Autodesk Inventor part; units mm, degrees
ref_plane "Work Plane2" through (0, 0, 20.5) normal (0, 0, 1) x (1, 0, 0)
ref_plane "YZ Plane" through (0, 0, 0) normal (1, 0, 0) x (0, 1, 0)
ref_plane "XZ Plane" through (0, 0, 0) normal (0, 1, 0) x (-1, 0, 0)
sketch "Sketch1" plane through (0, 0, 0) normal (0, 0, 1) x (1, 0, 0)
  circle A0 centre (0, 0) radius 20
  circle A1 centre (0, 15.55) radius 1.6
  line L0 (-20, 0) -> (20, 0) construction
  line L1 (20, 0) -> (20, -42)
  line L2 (20, -42) -> (-20, -42)
  line L3 (-20, -42) -> (-20, 0)
  circle A2 centre (-13.4667, 7.775) radius 1.6
  circle A3 centre (-13.4667, -7.775) radius 1.6
  circle A4 centre (0, -15.55) radius 1.6
  circle A5 centre (13.4667, -7.775) radius 1.6
  circle A6 centre (13.4667, 7.775) radius 1.6
  line L4 (0, -7) -> (0, 7) construction
  line L5 (-6.5, -7) -> (-6.5, 7)
  line L6 (6.5, 7) -> (6.5, -7)
  arc A7 (-6.5, -7) -> (6.5, -7) centre (0, -7) ccw
  arc A8 (6.5, 7) -> (-6.5, 7) centre (0, 7) ccw
  dimension "d0" = 40
  dimension "d1" = 15.55
  dimension "d3" = 42
  dimension "d6" = 360
  dimension "d8" = 6.5
  dimension "d9" = 14
extrude "Extrusion1" add sketch "Sketch1" along normal blind 7 contours A0 | L1 L2 L3 A0 | A1 | A2 | A3 | A4 | A5 | A6
sketch "Sketch2" plane through (0, 0, 0) normal (0, 0, -1) x (-1, 0, 0)
  line L0 (20, 0) -> (20, -42)
  arc A0 (20, 0) -> (-20, 0) centre (0, 0) ccw
  line L1 (-20, -42) -> (-20, 0)
  line L2 (20, -42) -> (-20, -42)
  line L3 (-6.5, 7) -> (-6.5, -7)
  arc A1 (6.5, 7) -> (-6.5, 7) centre (0, 7) ccw
  line L4 (6.5, -7) -> (6.5, 7)
  arc A2 (-6.5, -7) -> (6.5, -7) centre (0, -7) ccw
  circle A3 centre (0, 0) radius 15.5 construction
  circle A4 centre (-7.75, 13.4234) radius 1.6
  line L5 (0, 0) -> (-7.75, 13.4234) construction
  line L6 (0, 0) -> (0, 15.5) construction
  circle A5 centre (-15.5, 0) radius 1.6
  circle A6 centre (-7.75, -13.4234) radius 1.6
  circle A7 centre (7.75, -13.4234) radius 1.6
  circle A8 centre (15.5, 0) radius 1.6
  circle A9 centre (7.75, 13.4234) radius 1.6
  dimension "d12" = 31
  dimension "d13" = 3.2
  dimension "d14" = 30
  dimension "d17" = 360
extrude "Extrusion2" cut sketch "Sketch2" against normal through all contours A4 | A5 | A6 | A7 | A8 | A9
sketch "Sketch3" plane through (-20, -42, 0) normal (0, -1, 0) x (1, 0, 0)
  line L0 (0, 0) -> (40, 0)
  line L1 (40, 0) -> (40, 7)
  line L2 (0, 7) -> (40, 7)
  line L3 (0, 0) -> (0, 7)
  line L4 (40, 0) -> (40, 7)
  line L5 (40, 7) -> (0, 7)
  line L6 (0, 7) -> (0, 40)
  line L7 (0, 40) -> (40, 40)
  line L8 (40, 40) -> (40, 7)
  point P0 (20, 0)
  dimension "d21" = 40
extrude "Extrusion3" add sketch "Sketch3" against normal blind 8 contours L6 L7 L8 L2
fillet "Fillet1" radius 2 1 edges at (0, -42, 0)
sketch "Sketch4" plane through (-20, -42, 2) normal (0, -1, 0) x (1, 0, 0)
  line L0 (40, 38) -> (0, 38)
  line L1 (0, 0) -> (0, 38)
  line L2 (40, 0) -> (0, 0)
  line L3 (40, 0) -> (40, 38)
  line L4 (5, 4) -> (-5, 4)
  line L5 (-5, 4) -> (-5, 11)
  line L6 (-5, 11) -> (5, 11)
  line L7 (5, 11) -> (5, 4)
  line L8 (5, 4) -> (-5, 11) construction
  line L9 (-5, 4) -> (5, 11) construction
  circle A0 centre (-5, 7.5) radius 3.5
  circle A1 centre (-5, 7.5) radius 1.75
  point P0 (20, -2)
  point P1 (0, 7.5)
  point P2 (0, 4)
  point P3 (0, 11)
  point P4 (-5, 11)
  dimension "d26" = 7
  dimension "d27" = 5
  dimension "d28" = 4
  dimension "d29" = 3.5
extrude "Extrusion4" add sketch "Sketch4" against normal blind 4 contours L1 L4 A0 L6 | A0 L5 A1 | L5 A1 A0
ref_plane "Work Plane1" through (0, 0, 22.5) normal (0, 0, 1) x (1, 0, 0)
ref_plane "Work Plane2" through (0, 0, 20.5) normal (0, 0, 1) x (1, 0, 0)
mirror "Mirror2" about plane through (0, 0, 0) normal (1, 0, 0) of "Extrusion4"
mirror "Mirror3" about plane through (0, 0, 20.5) normal (0, 0, 1) of "Extrusion4", "Mirror2"
fillet "Fillet4" radius 2 8 edges at (20, -40, 6) (20, -40, 28) (-20, -40, 6) (-20, -40, 13) (-20, -40, 28) (-20, -40, 35) (20, -40, 35) (20, -40, 13)
properties part number "08_Ga_dong_co_02" material "Polyethylene, High Density"
Geometry check sheet. Reference: the model listing, model coordinates, mm. A direction names the side the tool comes from. Coordinates: 2 decimals unless noted, no trailing zeros. Loops run counter-clockwise (first coordinate to the right, second up) from the corner with the lowest first, then second, coordinate; pieces in that order, holes last.
Item 1: Access from +Z, -Z, +X, -X, +Y, -Y to the whole of each face (thin tool, end or side, straight path). Record for faces 4 (the face through (-5, -13, 7)), 5 (the face through (24, -40, 6)), 6 (the face through (0.1, -13.5, 3.5)), 7 (the face through (-20, -27.3, 6.6)).
Item 2: Sectioned sample at A-A, the plane z = 31.5. Record the boundary of the cut face in (x, y), then the cut area to 3 significant figures.
Item 3: Sectioned sample at C-C, the plane x = -7.75. Record the boundary of the cut face in (y, z), then the cut area to 3 significant figures.
Item 4: Release check for a two-part mould opening along Z. For faces 1 (the face through (23, -38, 10)), 2 (the face through (26.75, -40.03, 9.42)), 3 (the face through (-23, -40, 6)) record: released by +Z, released by -Z, zero draft, split by the parting line, or undercut.
Item 5: Sectioned sample at D-D, the plane y = -32.5. Record the boundary of the cut face in (x, z), then the cut area to 3 significant figures.
Item 6: Thickness scan on line 1 (X direction, y = -39.4, z = 9.5); line 2 (Z direction, x = 25, y = -39); line 3 (Y direction, x = 7.75, z = 2.5). Record the ranges inside material, lowest first.
Item 7: Go/stop test with flat-tipped pins: pin 1 Ø1 at (x, z) = (-4, 10) entering from +Y; pin 2 Ø8 at (y, z) = (-35, 23.5) entering from +X; pin 3 Ø4 at (x, z) = (-23.5, 11.5) entering from +Y. Record where each tip stops, or that it passes through.
Item 8: Sectioned sample at B-B, the plane x = 0. Record the boundary of the cut face in (y, z).
Check result:
1. face 4: +Z, +X, -X, +Y
1. face 5: -Z, +X, +Y, -Y
1. face 6: +Z, -Z
1. face 7: -X, +Y
2. outline: (-28.5, -42) - (-26.75, -42) - (-26.75, -38) - (-28.5, -38) - close; (-23.25, -42) - (23.25, -42) - (23.25, -38) - (20, -38) - (20, -34) - (-20, -34) - (-20, -38) - (-23.25, -38) - close; (26.75, -42) - (28.5, -42) - (28.5, -38) - (26.75, -38) - close
2. area: 360 mm2
3. outline: (-42, 2) arc R2 ccw to (-40, 0) - (-15.02, 0) - (-15.02, 7) - (-34, 7) - (-34, 40) - (-42, 40) - close; (-11.82, 0) - (11.82, 0) - (11.82, 7) - (-11.82, 7) - close; (15.02, 0) - (18.44, 0) - (18.44, 7) - (15.02, 7) - close
3. area: 641 mm2
4. face 1: zero draft
4. face 2: undercut
4. face 3: released by -Z
5. outline: (-20, 0) - (20, 0) - (20, 7) - (-20, 7) - close
5. area: 280 mm2
6. line 1: x = -28.5 to -26.75, -23.25 to 23.25, 26.75 to 28.5
6. line 2: z = 6 to 7.75, 11.25 to 13, 28 to 29.75, 33.25 to 35
6. line 3: y = -42 to -15.02, -11.82 to 11.82, 15.02 to 18.44
7. pin 1: stops at y = -34
7. pin 2: stops at x = 20.01
7. pin 3: stops at y = -38
8. outline: (-42, 2) arc R2 ccw to (-40, 0) - (-13.5, 0) - (-13.5, 7) - (-34, 7) - (-34, 40) - (-42, 40) - close; (13.5, 0) - (20, 0) - (20, 7) - (13.5, 7) - close
